```python
from build123d import *

# Parameters (mm, degrees)
SKETCH1_R            = 1.5875
BOSS_EXTRUDE1_DEPTH  = 2
BOSS_EXTRUDE2_START  = -2
BOSS_EXTRUDE2_DEPTH  = 5
BOSS_EXTRUDE3_START  = 1
SKETCH2_R            = 2.5
SKETCH2_R_2          = 1.5875
BOSS_EXTRUDE3_DEPTH  = 1
BOSS_EXTRUDE4_START  = -2
SKETCH1_4_W          = 4.25
SKETCH1_4_H          = 0.34
BOSS_EXTRUDE4_DEPTH  = 3
SKETCH3_R            = 1.5875
BOSS_EXTRUDE5_DEPTH  = 3
M3_CLEARANCE_HOLE1_D = 3.2


with BuildPart() as part:
    # Sketch1 → Boss-Extrude1 (new body)
    with BuildSketch(Plane(origin=(0, 0, 0), x_dir=(1, 0, 0), z_dir=(0, 1, 0))):
        Polygon((-10.42, 55.34), (-10.42, -2), (28.09, -2), (28.09, -0.34), (32.34, -0.34), (32.34, -2), (68.04, -2), (68.04, 12.125572875), (70.58, 14.665572875), (70.58, 49.088427125), (68.04, 51.628427125), (68.04, 55.34), (32.34, 55.34), (32.34, 57), (28.09, 57), (28.09, 55.34), align=None)
        with Locations(Location((15.24, 2.54, 0), (0, 0, 270))):
            Circle(SKETCH1_R, mode=Mode.SUBTRACT)
        with Locations(Location((66.04, 45.72, 0), (0, 0, 270))):
            Circle(SKETCH1_R, mode=Mode.SUBTRACT)
        with Locations(Location((13.97, 50.8, 0), (0, 0, 270))):
            Circle(SKETCH1_R, mode=Mode.SUBTRACT)
        with Locations(Location((66.04, 17.78, 0), (0, 0, 270))):
            Circle(SKETCH1_R, mode=Mode.SUBTRACT)
    extrude(amount=-BOSS_EXTRUDE1_DEPTH)

    # Sketch1<3> → Boss-Extrude2 (add)
    with BuildSketch(Plane(origin=(0, 0, 0), x_dir=(1, 0, 0), z_dir=(0, 1, 0)).offset(BOSS_EXTRUDE2_START)):
        Polygon((28.09, 55.34), (-2, 55.34), (-2, -2), (28.09, -2), (28.09, 0), (0, 0), (0, 53.34), (66.04, 53.34), (66.04, 50.8), (68.58, 48.26), (68.58, 15.494), (66.04, 12.954), (66.04, 0), (32.34, 0), (32.34, -2), (68.04, -2), (68.04, 12.125572875), (70.58, 14.665572875), (70.58, 49.088427125), (68.04, 51.628427125), (68.04, 55.34), (32.34, 55.34), (32.34, 57), (28.09, 57), align=None)
    extrude(amount=-BOSS_EXTRUDE2_DEPTH)

    # Sketch2 → Boss-Extrude3 (add)
    # profile 1 of 6: a face of its own
    with BuildSketch(Plane(origin=(0, 0, 0), x_dir=(1, 0, 0), z_dir=(0, 1, 0)).offset(BOSS_EXTRUDE3_START)):
        with Locations(Location((13.97, 50.8, 0), (0, 0, 270))):
            Circle(SKETCH2_R)
        with Locations(Location((13.97, 50.8, 0), (0, 0, 270))):
            Circle(SKETCH2_R_2, mode=Mode.SUBTRACT)
    # profile 2 of 6: a face of its own
    with BuildSketch(Plane(origin=(0, 0, 0), x_dir=(1, 0, 0), z_dir=(0, 1, 0)).offset(BOSS_EXTRUDE3_START)):
        with Locations(Location((66.04, 45.72, 0), (0, 0, 270))):
            Circle(SKETCH2_R)
        with Locations(Location((66.04, 45.72, 0), (0, 0, 270))):
            Circle(SKETCH2_R_2, mode=Mode.SUBTRACT)
    # profile 3 of 6: a face of its own
    with BuildSketch(Plane(origin=(0, 0, 0), x_dir=(1, 0, 0), z_dir=(0, 1, 0)).offset(BOSS_EXTRUDE3_START)):
        with Locations(Location((66.04, 17.78, 0), (0, 0, 270))):
            Circle(SKETCH2_R)
        with Locations(Location((66.04, 17.78, 0), (0, 0, 270))):
            Circle(SKETCH2_R_2, mode=Mode.SUBTRACT)
    # profile 4 of 6: a face of its own
    with BuildSketch(Plane(origin=(0, 0, 0), x_dir=(1, 0, 0), z_dir=(0, 1, 0)).offset(BOSS_EXTRUDE3_START)):
        with Locations(Location((15.24, 2.54, 0), (0, 0, 270))):
            Circle(SKETCH2_R)
        with Locations(Location((15.24, 2.54, 0), (0, 0, 270))):
            Circle(SKETCH2_R_2, mode=Mode.SUBTRACT)
    # profile 5 of 6: a face of its own
    with BuildSketch(Plane(origin=(0, 0, 0), x_dir=(1, 0, 0), z_dir=(0, 1, 0)).offset(BOSS_EXTRUDE3_START)):
        with Locations(Location((-6.21, 2.21, 0), (0, 0, 270))):
            Circle(SKETCH2_R)
    # profile 6 of 6: a face of its own
    with BuildSketch(Plane(origin=(0, 0, 0), x_dir=(1, 0, 0), z_dir=(0, 1, 0)).offset(BOSS_EXTRUDE3_START)):
        with Locations(Location((-6.21, 51.13, 0), (0, 0, 270))):
            Circle(SKETCH2_R)
    extrude(amount=-BOSS_EXTRUDE3_DEPTH)

    # Sketch1<4> → Boss-Extrude4 (add)
    with BuildSketch(Plane(origin=(0, 0, 0), x_dir=(1, 0, 0), z_dir=(0, 1, 0)).offset(BOSS_EXTRUDE4_START)):
        with Locations((30.215, -0.17)):
            Rectangle(SKETCH1_4_W, SKETCH1_4_H)
        Polygon((26.44, 0), (28.09, 0), (32.34, 0), (33.99, 0), (33.99, 1.31), (26.44, 1.31), align=None)
    extrude(amount=-BOSS_EXTRUDE4_DEPTH)

    # Sketch3 → Boss-Extrude5 (add)
    # profile 1 of 4: a face of its own
    with BuildSketch(Plane.XZ.offset(2)):
        with BuildLine():
            Line((12.74, 0), (12.74, -2.54))
            ThreePointArc((12.74, -2.54), (15.24, -5.04), (17.74, -2.54))
            Line((17.74, -2.54), (17.74, 0))
            Line((17.74, 0), (12.74, 0))
        make_face()
        with Locations(Location((15.24, -2.54, 0), (0, 0, 90))):
            Circle(SKETCH3_R, mode=Mode.SUBTRACT)
    # profile 2 of 4: a face of its own
    with BuildSketch(Plane.XZ.offset(2)):
        with BuildLine():
            Line((16.47, -53.34), (16.47, -50.8))
            ThreePointArc((16.47, -50.8), (13.97, -48.3), (11.47, -50.8))
            Line((11.47, -50.8), (11.47, -53.34))
            Line((11.47, -53.34), (16.47, -53.34))
        make_face()
        with Locations(Location((13.97, -50.8, 0), (0, 0, 90))):
            Circle(SKETCH3_R, mode=Mode.SUBTRACT)
    # profile 3 of 4: a face of its own
    with BuildSketch(Plane.XZ.offset(2)):
        with BuildLine():
            Line((68.58, -48.22), (66.04, -48.22))
            ThreePointArc((66.04, -48.22), (63.54, -45.72), (66.04, -43.22))
            Line((66.04, -43.22), (68.58, -43.22))
            Line((68.58, -43.22), (68.58, -48.22))
        make_face()
        with Locations(Location((66.04, -45.72, 0), (0, 0, 90))):
            Circle(SKETCH3_R, mode=Mode.SUBTRACT)
    # profile 4 of 4: a face of its own
    with BuildSketch(Plane.XZ.offset(2)):
        with BuildLine():
            Line((68.58, -20.28), (66.04, -20.28))
            ThreePointArc((66.04, -20.28), (63.54, -17.78), (66.04, -15.28))
            Line((66.04, -15.28), (68.58, -15.28))
            Line((68.58, -15.28), (68.58, -20.28))
        make_face()
        with Locations(Location((66.04, -17.78, 0), (0, 0, 90))):
            Circle(SKETCH3_R, mode=Mode.SUBTRACT)
    extrude(amount=BOSS_EXTRUDE5_DEPTH)

    # M3 Clearance Hole1 (through all)
    with Locations(Plane(origin=(0, 1, 0), x_dir=(1, 0, 0), z_dir=(0, 1, 0))):
        with Locations((-6.21, 51.13), (-6.21, 2.21)):
            Hole(M3_CLEARANCE_HOLE1_D / 2)


solid = part.part
```
Could you check a few things on this model? Use its own coordinates, in mm. A direction names the side the tool comes from. Give positions to 0.01 mm unless a question says otherwise; leave off trailing zeros. Loops run counter-clockwise (first coordinate to the right, second up) from the corner with the lowest first, then second, coordinate; pieces in that order, holes last. Notation, with made-up numbers: (39, 30.25) - (54, 30.25) arc R18 cw to (54, 44.25) - close; hole circle Ø11 at (66, -35). An arc over 180 degrees is marked (long way). Use one line per item in the form item = value.
1. I want a section at D-D (y = -3.5). Give the number of separate pieces and of enclosed holes in the cut face, and give its area (3 significant figures).
Response values:
separate_pieces = 1
enclosed_holes = 5
area = 566 mm²
2. Thinking about a two-plate mould opening in Z: for faces 1 (the face through (-2, -4, -27)), 2 (the face through (63.54, -3.48, -45.77)), 3 (the face through (16.47, -3, -52)), 4 (the face through (50, -3, -55.34)), which applies, released by +Z, released by -Z, zero draft, split by the parting line, or undercut?
Response values:
face_1 = zero draft
face_2 = undercut
face_3 = undercut
face_4 = released by -Z
3. I need wall thicknesses on probe 1 along Z at (x, y) = (66.04, -1.3); probe 2 along Z at (x, y) = (-6.21, -0.55); probe 3 along Z at (x, y) = (0.5, -5.25). Which ranges of each line are inside material? Lowest first, please.
Response values:
probe_1 = -55.34 to -47.31, -44.13 to -19.37, -16.19 to 2
probe_2 = -55.34 to -52.73, -49.53 to -3.81, -0.61 to 2
probe_3 = -55.34 to -53.34, 0 to 2
4. I want a section at C-C (z = -26). Please give me the cut outline in (x, y).
Response values:
outline = (-10.42, -2) - (-2, -2) - (-2, -7) - (0, -7) - (0, -2) - (68.58, -2) - (68.58, -7) - (70.58, -7) - (70.58, 0) - (-10.42, 0) - close
5. I'm going to push flat-ended pins straight in: pin 1 Ø3 at (x, y) = (47, -2) entering from -Z; pin 2 Ø8 at (x, z) = (41, -46) entering from -Y; pin 3 Ø4 at (x, z) = (66.04, -17.78) entering from -Y. Where does each tip first touch, or does it pass through?
Response values:
pin_1 = -55.34
pin_2 = -2
pin_3 = -5
6. I want a section at B-B (z = -17.78). Please give me the cut outline in (x, y), and give its area (3 significant figures).
Response values:
outline = (-10.42, -2) - (-2, -2) - (-2, -7) - (0, -7) - (0, -2) - (63.54, -2) - (63.54, -5) - (64.45, -5) - (64.45, 1) - (63.54, 1) - (63.54, 0) - (-10.42, 0) - close; (67.63, -5) - (68.58, -5) - (68.58, -7) - (70.58, -7) - (70.58, 0) - (68.54, 0) - (68.54, 1) - (67.63, 1) - close
area = 183 mm²
7. On a 3-axis mill with a long thin cutter (end or side, diameter ignored), from which of +Z, -Z, +X, -X, +Y, -Y can I reach the whole of each face in a straight line? I mean faces 5 (the face through (68.04, -3, -5)), 6 (the face through (70.58, -3, -32)), 7 (the face through (68, -5, -46)), 8 (the face through (-6.1, 0.507, -53.628)). Say none if no direction works.
Response values:
face_5 = +Z, +X, +Y, -Y
face_6 = +Z, -Z, +X, +Y, -Y
face_7 = -Y
face_8 = +Y
8. I want a section at A-A (x = -6.21). Please give me the cut outline in (y, z).
Response values:
outline = (-2, -55.34) - (0, -55.34) - (0, -53.63) - (1, -53.63) - (1, -52.73) - (-2, -52.73) - close; (-2, -49.53) - (1, -49.53) - (1, -48.63) - (0, -48.63) - (0, -4.71) - (1, -4.71) - (1, -3.81) - (-2, -3.81) - close; (-2, -0.61) - (1, -0.61) - (1, 0.29) - (0, 0.29) - (0, 2) - (-2, 2) - close
